Read the model definition and answer for the solid it produces. Units are mm, in the model's axes. A direction names the side the tool comes from. Round coordinates to 2 decimals unless told otherwise and drop trailing zeros. Order: outer loops, then holes, each group sorted by start corner. A loop starts at its lowest first (then second) coordinate and runs counter-clockwise, first axis right, second up. Notation, with made-up numbers: (13.25, 19) -> (27.25, 19) arc R21 ccw to (27.25, 37) -> close; hole circle Ø8 at (76, 78). An arc over 180 degrees is marked (long way). Answer as a JSON object with one key per item and string values. Group by question number.
Item 1: For faces 1 (the flat face through (124.5, 18, 2)), 2 (the flat face through (-124.5, -17, 2)), 3 (the flat face through (124.5, -18, 2)), 4 (the flat face through (-124.5, 17, 2)), determine the directions among +Z, -Z, +X, -X, +Y, -Y from which every point of the face is accessible in a straight line to the end or side of a thin tool.
Item 2: Section B-B, the plane x = -127.5 is taken. Write down the section's boundary in (y, z), plus the area to 3 significant figures.
Item 3: Consider probe 1 along Y at (x, z) = (-128.5, 0.25); probe 2 along X at (y, z) = (-15.5, 1.7). Determine where each line is inside the solid, lowest interval first. Write a range as from..to.
Item 4: Section A-A, the plane z = 4.2 is taken. Write down the section's boundary in (x, y), plus the area to 3 significant figures.
Item 5: Given P1, Ø1.5, axis at x = 137, z = 3, coming from the -Y side; P2, Ø1.5, axis at x = -139.5, z = 2.5, coming from the +Y side; P3, Ø2.5, axis at y = 16.5, z = 2, coming from the -X side, each flat-ended and moving along its own axis, determine where each tip first touches the part or whether it passes through.
Autodesk Inventor part; units mm, degrees
ref_plane "YZ Plane" through (0, 0, 0) normal (1, 0, 0) x (0, 1, 0)
ref_plane "XZ Plane" through (0, 0, 0) normal (0, 1, 0) x (-1, 0, 0)
ref_plane "XY Plane" through (0, 0, 0) normal (0, 0, 1) x (1, 0, 0)
sketch "Sketch1" plane through (0, 0, 0) normal (0, 0, 1) x (1, 0, 0)
  line L0 (-150, -15) -> (150, -15)
  line L1 (150, -15) -> (150, 15)
  line L2 (150, 15) -> (-150, 15)
  line L3 (-150, 15) -> (-150, -15)
  line L4 (-150, -15) -> (150, 15) construction
  line L5 (150, -15) -> (-150, 15) construction
  line L6 (-124.5, 20) -> (124.5, 20)
  line L7 (124.5, 20) -> (124.5, 15)
  line L8 (124.5, 15) -> (-124.5, 15)
  line L9 (-124.5, 15) -> (-124.5, 20)
  line L10 (-124.5, 20) -> (124.5, 15) construction
  line L11 (124.5, 20) -> (-124.5, 15) construction
  line L12 (-150, 0) -> (150, 0)
  line L13 (-124.5, -20) -> (124.5, -20)
  line L14 (124.5, -20) -> (124.5, -15)
  line L15 (124.5, -15) -> (-124.5, -15)
  line L16 (-124.5, -15) -> (-124.5, -20)
  line L17 (-124.5, -20) -> (124.5, -15) construction
  line L18 (124.5, -20) -> (-124.5, -15) construction
  point P0 (0, 0)
  point P1 (0, 0)
  point P2 (0, 17.5)
  point P3 (0, 15)
  point P4 (-77.3047, 14.0744)
  point P5 (81.6953, 14.0744)
  point P6 (0, -15)
  point P7 (0, -17.5)
  dimension "d0" = 5
  dimension "d1" = 30
  dimension "d2" = 300
  dimension "d3" = 249
extrude "Plate1" add sketch "Sketch1" along normal blind 5
equation "\"d4\" = Thickness"
equation "\"BendRadius\" = Thickness"
equation "\"BendReliefWidth\" = Thickness"
equation "\"BendReliefDepth\" = 0.5 * Thickness"
equation "\"TransitionRadius\" = BendRadius"
equation "\"JacobiRadiusSize\" = BendRadius"
equation "\"GapSize\" = Thickness"
properties part number "Base Leg V2"
Values found:
{
 "1": {"face 1": "+Z, -Z, +X, +Y", "face 2": "+Z, -Z, -X, -Y", "face 3": "+Z, -Z, +X, -Y", "face 4": "+Z, -Z, -X, +Y"},
 "2": {"outline": "(-15, 0) -> (15, 0) -> (15, 5) -> (-15, 5) -> close", "area": "150 mm2"},
 "3": {"probe 1": "-15..15", "probe 2": "-124.5..124.5"},
 "4": {"outline": "(-150, -15) -> (-124.5, -15) -> (-124.5, -20) -> (124.5, -20) -> (124.5, -15) -> (150, -15) -> (150, 15) -> (124.5, 15) -> (124.5, 20) -> (-124.5, 20) -> (-124.5, 15) -> (-150, 15) -> close", "area": "11,500 mm2"},
 "5": {"P1": "y = -15", "P2": "y = 15", "P3": "x = -124.5"}
}
